CAD build for the part. Positions are in the model's coordinates, mm. A direction names the side the tool comes from. Coordinates: 2 decimals unless noted, no trailing zeros. Order: outer loops, then holes, each group sorted by start corner. A loop starts at its lowest first (then second) coordinate and runs counter-clockwise, first axis right, second up. Notation, with made-up numbers: (52.5, -16) - (67.5, -16) arc R31 cw to (67.5, 21) - close; hole circle Ø5 at (-27, 89). An arc over 180 degrees is marked (long way). Return JSON: item names as keys, results as strings.
from build123d import *

# Parameters (mm, degrees)
F1_DEPTH = 12.7
F3_DEPTH = 7.62
F5_DEPTH = 25.4
F7_DEPTH = 25.4


with BuildPart() as f1:
    # F0 (on Top) → F1 (new body)
    with BuildSketch(Plane.XY):
        Polygon((0.824413, 28.39133), (-5.525587, 8.07133), (7.174413, 8.07133), align=None)
    extrude(amount=F1_DEPTH)

    # F2 (on face) → F3 (join)
    with BuildSketch(Plane(origin=(0, 0, 0), x_dir=(1, 0, 0), z_dir=(0, 0, -1))):
        Polygon((2.094413, -24.32733), (-0.445587, -24.32733), (0.824413, -28.39133), align=None)
    extrude(amount=F3_DEPTH)

    # F4 (on face) → F5 (cut)
    with BuildSketch(Plane(origin=(-7.331874, 2.291211, 0), x_dir=(-0.298275, -0.95448, 0), z_dir=(-0.95448, 0.298275, 0))):
        Polygon((-23.087042, -7.62), (-23.087042, 0), (-27.344858, -7.62), align=None)
    extrude(amount=-F5_DEPTH, mode=Mode.SUBTRACT)

    # F6 (on face) → F7 (cut)
    with BuildSketch(Plane(origin=(8.834008, 2.760627, 0), x_dir=(-0.298275, 0.95448, 0), z_dir=(0.95448, 0.298275, 0))):
        Polygon((26.853055, -7.62), (22.595239, 0), (22.595239, -1.355872), align=None)
    extrude(amount=-F7_DEPTH, mode=Mode.SUBTRACT)


solid = f1.part
Item 1: Drop flat-ended pins along their axis: P1, Ø10, axis at y = 18.5, z = 5, coming from the +X side; P2, Ø5, axis at x = -1, y = 24.5, coming from the -Z side; P3, Ø1, axis at x = 0, y = 12, coming from the -Z side. Give the stop position or say it passes through.
Findings below:
{"P1": "stops at x = 5.48", "P2": "stops at z = -4.35", "P3": "stops at z = 0"}
Item 2: Band-saw the part on A-A, the plane x = 0.5. List the corners of the cut face in (y, z), then the cut area to 3 significant figures.
Findings below:
{"outline": "(8.07, 0) - (24.33, 0) - (24.33, -0.5) - (27.35, -5.67) - (27.35, 12.7) - (8.07, 12.7) - close", "area": "254 mm²"}
Item 3: Which spindle directions (+Z, -Z, +X, -X, +Y, -Y) get a long thin tool onto all of the face, cutting with end or side? Do faces 4 (the flat face through (1, 15, 0)), 5 (the flat face through (1, 16, 12.7)). Say none if no direction does.
Findings below:
{"face 4": "-Z, +X, -X, -Y", "face 5": "+Z, +X, -X, +Y, -Y"}
Item 4: Band-saw the part on C-C, the plane y = 16. List the corners of the cut face in (x, z).
Findings below:
{"outline": "(-3.05, 0) - (4.7, 0) - (4.7, 12.7) - (-3.05, 12.7) - close"}
Item 5: Mould opens along X. For faces 1 (the flat face through (1, 8.071, 6)), 2 (the flat face through (-2.395, 18.089, 4.94)), 3 (the flat face through (3.955, 18.374, 4.94)) say: released by +X, released by -X, zero draft, split by the parting line, or undercut.
Findings below:
{"face 1": "zero draft", "face 2": "released by -X", "face 3": "released by +X"}
Item 6: Band-saw the part on D-D, the plane x = -3. List the corners of the cut face in (y, z), then the cut area to 3 significant figures.
Findings below:
{"outline": "(8.07, 0) - (16.15, 0) - (16.15, 12.7) - (8.07, 12.7) - close", "area": "103 mm²"}
Item 7: Band-saw the part on B-B, the plane z = 10.25. List the corners of the cut face in (x, y).
Findings below:
{"outline": "(-5.53, 8.07) - (7.17, 8.07) - (0.82, 28.39) - close"}
Item 8: Wall check: L1, parallel to Z at x = -1.75, y = 17.25; L2, parallel to X at y = 19.5, z = 1.25; L3, parallel to X at y = 22.5, z = 6.5. Give the ranges that are in metal, low to high. Write a range as [from, to].
Findings below:
{"L1": "z = [0, 12.7]", "L2": "x = [-1.95, 3.6]", "L3": "x = [-1.02, 2.67]"}
